Geometry: final body of the model. Coordinates: model frame, mm. Give positions to 0.01 mm unless a question says otherwise; leave off trailing zeros. Write each loop counter-clockwise with the first axis right and the second up, starting at its lowest first coordinate (ties: lowest second). Pieces come first, ordered by that corner, then holes. Notation, with made-up numbers: (45.5, 5) - (57.5, 5) arc R9 ccw to (57.5, 11) - close; hole circle Ø4 at (22.25, -28). An arc over 180 degrees is marked (long way). Return JSON: item names as keys, results as strings.
from build123d import *

# Parameters (mm, degrees)
F0_W     = 215.9
F0_H     = 101.6
F0_R     = 2.579688
F0_R_2   = 1.389063
F0_R_3   = 3.373438
F1_DEPTH = 6.35
F2_SIZE  = 1.9812


with BuildPart() as f1:
    # F0 (on Top) → F1 (new body)
    with BuildSketch(Plane.XY):
        Rectangle(F0_W, F0_H)
        with Locations((-101.0031, -21.59)):
            Circle(F0_R, mode=Mode.SUBTRACT)
        with Locations((36.83, -40.64)):
            Circle(F0_R_2, mode=Mode.SUBTRACT)
        with Locations((62.23, -40.64)):
            Circle(F0_R_2, mode=Mode.SUBTRACT)
        with Locations((101.6, -44.45)):
            Circle(F0_R_2, mode=Mode.SUBTRACT)
        Circle(F0_R, mode=Mode.SUBTRACT)
        with Locations((-101.0031, 6.0579)):
            Circle(F0_R, mode=Mode.SUBTRACT)
        with Locations((-70.4469, 6.0579)):
            Circle(F0_R, mode=Mode.SUBTRACT)
        with Locations((-52.32654, 19.05)):
            Circle(F0_R_3, mode=Mode.SUBTRACT)
        with Locations((-101.0031, 32.0421)):
            Circle(F0_R, mode=Mode.SUBTRACT)
        with Locations((-70.4469, 32.0421)):
            Circle(F0_R, mode=Mode.SUBTRACT)
        with Locations((-15.875, 41.91)):
            Circle(F0_R, mode=Mode.SUBTRACT)
        with Locations((52.32654, 19.05)):
            Circle(F0_R_3, mode=Mode.SUBTRACT)
        with Locations((70.4469, 6.0579)):
            Circle(F0_R, mode=Mode.SUBTRACT)
        with Locations((101.0031, 6.0579)):
            Circle(F0_R, mode=Mode.SUBTRACT)
        with Locations((15.875, 41.91)):
            Circle(F0_R, mode=Mode.SUBTRACT)
        with Locations((70.4469, 32.0421)):
            Circle(F0_R, mode=Mode.SUBTRACT)
        with Locations((101.0031, 32.0421)):
            Circle(F0_R, mode=Mode.SUBTRACT)
    extrude(amount=F1_DEPTH)

    # F2
    f2_edges = [f1.edges().sort_by_distance(p)[0] for p in [
        (-73.026588, 32.0421, 6.35),
        (-103.582788, 32.0421, 6.35),
        (-103.582788, 6.0579, 6.35),
        (-73.026588, 6.0579, 6.35),
        (67.867212, 32.0421, 6.35),
        (67.867212, 6.0579, 6.35),
        (98.423412, 6.0579, 6.35),
        (98.423412, 32.0421, 6.35),
    ]]
    chamfer(f2_edges, length=F2_SIZE)


solid = f1.part
Q1. Mould query, pull axis X, two halves, no side actions, for faces 1 (the flat face through (107.95, -1, 3)), 2 (the flat face through (-107.95, -1, 3)), 3 (the conical face through (-73.148, 32.161, 4.493)). Classes: pulls with the +X half, pulls with the -X half, needs draft (parallel to the pull), parting line crosses it, or undercut.
Answer key:
{"face 1": "pulls with the +X half", "face 2": "pulls with the -X half", "face 3": "undercut"}
Q2. Section query B-B, the plane y = -21.59. Return the cut outline in (x, z).
Answer key:
{"outline": "(-107.95, 0) - (-103.58, 0) - (-103.58, 6.35) - (-107.95, 6.35) - close; (-98.42, 0) - (107.95, 0) - (107.95, 6.35) - (-98.42, 6.35) - close"}
Q3. Section query C-C, the plane x = -53. Return the cut outline in (y, z).
Answer key:
{"outline": "(-50.8, 0) - (15.74, 0) - (15.74, 6.35) - (-50.8, 6.35) - close; (22.36, 0) - (50.8, 0) - (50.8, 6.35) - (22.36, 6.35) - close"}
Q4. Section query D-D, the plane z = 1.25. Count the separate pieces of the cut face and the enclosed holes in it, plus the area to 3 significant figures.
Answer key:
{"separate pieces": "1", "enclosed holes": "17", "area": "21,600 mm^2"}
Q5. Material intervals for probe 1 along X at (y, z) = (30, 1.5); probe 2 along Y at (x, z) = (62.23, 2.5); probe 3 along Y at (x, z) = (-69, 5), sorted ascending. Write a range as [from, to].
Answer key:
{"probe 1": "x = [-107.95, -102.58], [-99.43, -72.02], [-68.87, 68.87], [72.02, 99.43], [102.58, 107.95]", "probe 2": "y = [-50.8, -42.03], [-39.25, 50.8]", "probe 3": "y = [-50.8, 3.19], [8.92, 29.18], [34.91, 50.8]"}
Q6. Pin query (flat end, axial travel): P1, Ø3, axis at x = -70.45, y = 32.04, coming from the +Z side; P2, Ø6.5, axis at x = 70.45, y = 6.06, coming from the +Z side. Return the tip coordinate at first contact, or that it passes through.
Answer key:
{"P1": "passes through", "P2": "stops at z = 5.04"}
Q7. Section query A-A, the plane y = 41.91. Return the cut outline in (x, z).
Answer key:
{"outline": "(-107.95, 0) - (-18.45, 0) - (-18.45, 6.35) - (-107.95, 6.35) - close; (-13.3, 0) - (13.3, 0) - (13.3, 6.35) - (-13.3, 6.35) - close; (18.45, 0) - (107.95, 0) - (107.95, 6.35) - (18.45, 6.35) - close"}
